Check sheet for the modelled part. Datum: model origin and axes. Units: mm. A direction names the side the tool comes from. Give positions to 0.01 mm unless a question says otherwise; leave off trailing zeros. Write each loop counter-clockwise with the first axis right and the second up, starting at its lowest first coordinate (ties: lowest second). Pieces come first, ordered by that corner, then holes. Notation, with made-up numbers: M 20.5,19.5 L 51.5,19.5 A24 ccw 51.5,39.5 Z; hole C -0.5,5 d11. An arc over 180 degrees is marked long. Write item = value, one per line. Start each with the question number.
1) Gauge pin test, flat ends, axial feed: pin 1 (2 mm diameter, centred on x = 2, z = 1, fed in from -Y); pin 2 (2 mm diameter, centred on y = -13.5, z = 1, fed in from -X); pin 3 (12 mm diameter, centred on x = 9.5, y = -7.5, fed in from -Z); pin 4 (0.6 mm diameter, centred on y = -32, z = 2, fed in from -X). Record the tip position at first contact, or that the pin passes through.
2) Sectioned sample at C-C, the plane x = 8. Record the cut outline in (y, z).
3) Draft check along X on faces 3 (the face through (-1, -8, 4)), 4 (the face through (-31.812, -17, 2)), 5 (the face through (-8, -22.478, 2)). Enter one of: pulls with the +X half, pulls with the -X half, needs draft (parallel to the pull), parting line crosses it, or undercut.
4) Set-up check for faces 1 (the face through (1.27, 20, 2)), 2 (the face through (-13.938, 34, 2)): record each of +Z, -Z, +X, -X, +Y, -Y from which the full face is reachable in a straight line by a thin tool's end or side.
5) Sectioned sample at B-B, the plane y = -4. Record the cut outline in (x, z).
6) Sectioned sample at A-A, the plane x = 0. Record the cut outline in (y, z), then the cut area to 3 significant figures.
7) Scan lines: L1, parallel to Y at x = 0, z = 2.1; L2, parallel to X at y = 5.5, z = 1.05; L3, parallel to Y at x = 1.5, z = 3.2. Record each from-to range of solid material in increasing order.
8) Sectioned sample at D-D, the plane z = 3.2. Count the separate pieces of the cut face and the enclosed holes in it, then the cut area to 3 significant figures.
from build123d import *

# Parameters (mm, degrees)
SKETCH1_R           = 38.1
BOSS_EXTRUDE1_DEPTH = 4
SKETCH2_R           = 2.286
SKETCH2_W           = 12.7
SKETCH2_H           = 4
SKETCH2_W_2         = 4
SKETCH2_H_2         = 12.7
CUT_EXTRUDE1_DEPTH  = 55.029806589
CUT_EXTRUDE2_REACH  = 56.03
SKETCH3_W           = 12
SKETCH3_H           = 12.7
SKETCH4_R           = 1.9304
CUT_EXTRUDE3_DEPTH  = 55.029806589
CUT_EXTRUDE4_REACH  = 56.03
SKETCH5_W           = 5.08
SKETCH5_H           = 5.08


with BuildPart() as part:
    # Sketch1 → Boss-Extrude1 (new body)
    with BuildSketch(Plane.XY):
        Circle(SKETCH1_R)
    extrude(amount=BOSS_EXTRUDE1_DEPTH)

    # Sketch2 → Cut-Extrude1 (cut, through all)
    with BuildSketch(Plane.XY.offset(4)):
        with Locations((12.446, -29.464)):
            Circle(SKETCH2_R)
        with Locations((-29.464, -12.446)):
            Circle(SKETCH2_R)
        with Locations((-12.446, 29.464)):
            Circle(SKETCH2_R)
        with Locations((29.464, 12.446)):
            Circle(SKETCH2_R)
        with Locations((-7.62, -12.478)):
            Rectangle(SKETCH2_W, SKETCH2_H)
        with Locations((12.478, -7.62)):
            Rectangle(SKETCH2_W_2, SKETCH2_H_2)
        with Locations((20.478, -7.62)):
            Rectangle(SKETCH2_W_2, SKETCH2_H_2)
        with Locations((-7.62, -20.478)):
            Rectangle(SKETCH2_W, SKETCH2_H)
        with Locations((-12.478, 7.62)):
            Rectangle(SKETCH2_W_2, SKETCH2_H_2)
        with Locations((-20.478, 7.62)):
            Rectangle(SKETCH2_W_2, SKETCH2_H_2)
        with Locations((7.62, 12.478)):
            Rectangle(SKETCH2_W, SKETCH2_H)
        with Locations((7.62, 20.478)):
            Rectangle(SKETCH2_W, SKETCH2_H)
    extrude(amount=-CUT_EXTRUDE1_DEPTH, mode=Mode.SUBTRACT)

    # Sketch3 → Cut-Extrude2 (cut, up to next)
    with BuildSketch(Plane.XY.offset(4), mode=Mode.PRIVATE) as cut_extrude2_sk1:
        Rectangle(SKETCH3_W, SKETCH3_H)
    cut_extrude2_tool1 = extrude(cut_extrude2_sk1.sketch, amount=-CUT_EXTRUDE2_REACH, mode=Mode.PRIVATE) & part.part
    add(cut_extrude2_tool1.solids().sort_by_distance((0, 0, 4))[0], mode=Mode.SUBTRACT)

    # Sketch4 → Cut-Extrude3 (cut, through all)
    with BuildSketch(Plane.XY.offset(4)):
        with Locations((0, -31.75)):
            Circle(SKETCH4_R)
        with Locations((31.75, 0)):
            Circle(SKETCH4_R)
        with Locations((0, 31.75)):
            Circle(SKETCH4_R)
        with Locations((-31.75, 0)):
            Circle(SKETCH4_R)
    extrude(amount=-CUT_EXTRUDE3_DEPTH, mode=Mode.SUBTRACT)

    # Sketch5 → Cut-Extrude4 (cut, up to next)
    with BuildSketch(Plane.XY.offset(4), mode=Mode.PRIVATE) as cut_extrude4_sk1:
        with Locations((34.352372786, 16.478)):
            Rectangle(SKETCH5_W, SKETCH5_H)
    cut_extrude4_tool1 = extrude(cut_extrude4_sk1.sketch, amount=-CUT_EXTRUDE4_REACH, mode=Mode.PRIVATE) & part.part
    # Sketch5 → Cut-Extrude4 (cut, up to next)
    with BuildSketch(Plane.XY.offset(4), mode=Mode.PRIVATE) as cut_extrude4_sk2:
        with Locations((16.478, -34.352372786)):
            Rectangle(SKETCH5_W, SKETCH5_H)
    cut_extrude4_tool2 = extrude(cut_extrude4_sk2.sketch, amount=-CUT_EXTRUDE4_REACH, mode=Mode.PRIVATE) & part.part
    # Sketch5 → Cut-Extrude4 (cut, up to next)
    with BuildSketch(Plane.XY.offset(4), mode=Mode.PRIVATE) as cut_extrude4_sk3:
        with Locations((-34.352372786, -16.478)):
            Rectangle(SKETCH5_W, SKETCH5_H)
    cut_extrude4_tool3 = extrude(cut_extrude4_sk3.sketch, amount=-CUT_EXTRUDE4_REACH, mode=Mode.PRIVATE) & part.part
    # Sketch5 → Cut-Extrude4 (cut, up to next)
    with BuildSketch(Plane.XY.offset(4), mode=Mode.PRIVATE) as cut_extrude4_sk4:
        with Locations((-16.478, 34.352372786)):
            Rectangle(SKETCH5_W, SKETCH5_H)
    cut_extrude4_tool4 = extrude(cut_extrude4_sk4.sketch, amount=-CUT_EXTRUDE4_REACH, mode=Mode.PRIVATE) & part.part
    add(cut_extrude4_tool1.solids().sort_by_distance((34.352373, 16.478, 4))[0], mode=Mode.SUBTRACT)
    add(cut_extrude4_tool2.solids().sort_by_distance((16.478, -34.352373, 4))[0], mode=Mode.SUBTRACT)
    add(cut_extrude4_tool3.solids().sort_by_distance((-34.352373, -16.478, 4))[0], mode=Mode.SUBTRACT)
    add(cut_extrude4_tool4.solids().sort_by_distance((-16.478, 34.352373, 4))[0], mode=Mode.SUBTRACT)


solid = part.part
Data:
q1.pin_1 = -38.09
q1.pin_2 = -35.99
q1.pin_3 = 0
q1.pin_4 = -21.14
q2.outline = M -37.25,0 L 10.48,0 L 10.48,4 L -37.25,4 Z; M 14.48,0 L 18.48,0 L 18.48,4 L 14.48,4 Z; M 22.48,0 L 37.25,0 L 37.25,4 L 22.48,4 Z
q3.face_3 = needs draft
q3.face_4 = pulls with the -X half
q3.face_5 = undercut
q4.face_1 = +Z, -Z
q4.face_2 = +Z, -Z, +Y
q5.outline = M -37.89,0 L -6,0 L -6,4 L -37.89,4 Z; M 6,0 L 10.48,0 L 10.48,4 L 6,4 Z; M 14.48,0 L 18.48,0 L 18.48,4 L 14.48,4 Z; M 22.48,0 L 37.89,0 L 37.89,4 L 22.48,4 Z
q6.outline = M -38.1,0 L -33.68,0 L -33.68,4 L -38.1,4 Z; M -29.82,0 L -6.35,0 L -6.35,4 L -29.82,4 Z; M 6.35,0 L 29.82,0 L 29.82,4 L 6.35,4 Z; M 33.68,0 L 38.1,0 L 38.1,4 L 33.68,4 Z
q6.area = 223 mm2
q7.L1 = -38.1 to -33.68, -29.82 to -6.35, 6.35 to 29.82, 33.68 to 38.1
q7.L2 = -37.7 to -22.48, -18.48 to -14.48, -10.48 to -6, 6 to 37.7
q7.L3 = -38.07 to -32.97, -30.53 to -6.35, 6.35 to 10.48, 14.48 to 18.48, 22.48 to 30.53, 32.97 to 38.07
q8.separate_pieces = 1
q8.enclosed_holes = 17
q8.area = 3,840 mm2
